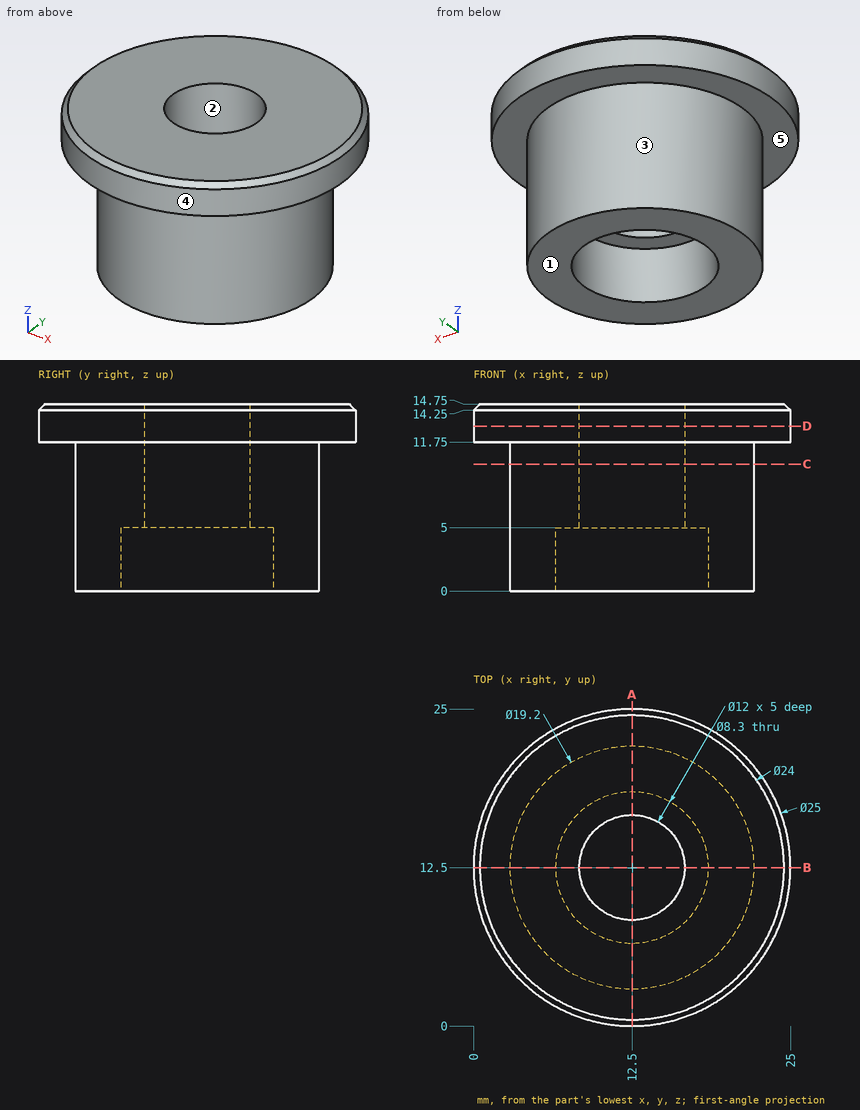
The figure shows three views and two pictorial views of one solid part (mm, origin at its lowest corner). Answer the questions. A direction names the side the tool comes from. Give positions to 0.01 mm unless a question says otherwise; leave off trailing zeros. Order: outer loops, then holes, each group sorted by start corner. A loop starts at its lowest first (then second) coordinate and runs counter-clockwise, first axis right, second up. Notation, with made-up numbers: (-12.5, 25) -> (31.5, 25) arc R13 cw to (31.5, 41) -> close; hole circle Ø8 at (78, 73.5). An arc over 180 degrees is marked (long way). Write each question's results on one line, items separated by ' | '.
Q1. The part is cut by section A-A, the plane x = 12.5. Give the vertices of the cut face in (y, z), and give its area (3 significant figures).
Checked values:
outline: (0, 11.75) -> (2.9, 11.75) -> (2.9, 0) -> (6.5, 0) -> (6.5, 5) -> (8.35, 5) -> (8.35, 14.75) -> (0.5, 14.75) -> (0, 14.25) -> close; (16.65, 5) -> (18.5, 5) -> (18.5, 0) -> (22.1, 0) -> (22.1, 11.75) -> (25, 11.75) -> (25, 14.25) -> (24.5, 14.75) -> (16.65, 14.75) -> close | area: 159 mm^2
Q2. The part is cut by section D-D, the plane z = 13. Give the vertices of the cut face in (x, y), and give its area (3 significant figures).
Checked values:
outline: circle Ø25 at (12.5, 12.5); hole circle Ø8.3 at (12.5, 12.5) | area: 437 mm^2
Q3. Straight lines are drawn through the part: probe 1 along Y at (x, z) = (12.5, 7.5); probe 2 along Y at (x, z) = (12.5, 1.9); probe 3 along Z at (x, y) = (2, 11.5). For each, find the intervals that lie inside material, in ascending order. Write a range as from..to.
Checked values:
probe 1: y = 2.9..8.35, 16.65..22.1 | probe 2: y = 2.9..6.5, 18.5..22.1 | probe 3: z = 11.75..14.75
Q4. Determine the mould class of the marked faces 1, 2 and 3 for opening direction X: pulls with the +X half, pulls with the -X half, needs draft (parallel to the pull), parting line crosses it, or undercut.
Checked values:
face 1: needs draft | face 2: undercut | face 3: parting line crosses it
Q5. Each of these flat-tipped pins is pushed along its axis until it touches: P1, Ø6, axis at x = 2.5, z = 9.5, coming from the +Y side; P2, Ø3, axis at x = 15.5, z = 5, coming from the +Y side; P3, Ø6, axis at x = 10, y = 12, coming from the -Z side; P4, Ø5, axis at x = 12.5, y = 12.5, coming from the -Z side. Where does it stop, or does it pass through?
Checked values:
P1: stops at y = 22.09 | P2: stops at y = 21.98 | P3: stops at z = 5 | P4: passes through
Q6. Which of the six approach directions +Z, -Z, +X, -X, +Y, -Y give full straight-line access (tool end or side, diameter ignored) to the marked faces 4 and 5?
Checked values:
face 4: +Z, -Z | face 5: -Z
Q7. The part is cut by section C-C, the plane z = 10. Give the vertices of the cut face in (x, y), and give its area (3 significant figures).
Checked values:
outline: circle Ø19.2 at (12.5, 12.5); hole circle Ø8.3 at (12.5, 12.5) | area: 235 mm^2
